Autodesk Inventor part; units mm, degrees
ref_plane "YZ Plane" through (0, 0, 0) normal (1, 0, 0) x (0, 1, 0)
ref_plane "XZ Plane" through (0, 0, 0) normal (0, 1, 0) x (-1, 0, 0)
ref_plane "XY Plane" through (0, 0, 0) normal (0, 0, 1) x (1, 0, 0)
sketch "Sketch1" plane through (0, 0, 0) normal (0, 0, 1) x (1, 0, 0)
  line L0 (0, 0) -> (66.675, 0)
  line L1 (66.675, 0) -> (66.675, 12.7)
  line L2 (66.675, 12.7) -> (0, 12.7)
  line L3 (0, 12.7) -> (0, 0)
  dimension "d0" = 66.675
  dimension "d1" = 12.7
extrude "Extrusion1" add sketch "Sketch1" along normal blind 5.08
fillet "Fillet1" radius 0.635 4 edges at (33.3375, 12.7, 0) (66.675, 6.35, 0) (33.3375, 0, 0) (0, 6.35, 0)
fillet "Fillet2" radius 0.635 8 edges at (66.489, 12.514, 0.186) (66.675, 12.7, 2.8575) (66.489, 0.186, 0.186) (66.675, 0, 2.8575) (0.186, 12.514, 0.186) (0, 12.7, 2.8575) (0.186, 0.186, 0.186) (0, 0, 2.8575)
sketch "Sketch2" plane through (0, 0, 5.08) normal (0, 0, 1) x (1, 0, 0)
  line L0 (9.525, 12.6996) -> (57.15, 12.6996)
  line L1 (57.15, 12.6996) -> (57.15, -0.0004)
  line L2 (57.15, -0.0004) -> (9.525, -0.0004)
  line L3 (9.525, -0.0004) -> (9.525, 12.6996)
  line L4 (66.675, 0.635) -> (66.675, 12.065)
  point P0 (0, 0)
  dimension "d6" = 47.625
  dimension "d7" = 12.7
  dimension "d8" = 9.525
extrude "Extrusion2" cut sketch "Sketch2" against normal blind 1.905
sketch "Sketch3" plane through (9.525, 12.6996, 5.08) normal (0, -1, 0) x (1, 0, 0)
  line L0 (0, -1.905) -> (0, 0)
  line L1 (47.625, -1.905) -> (0, -1.905)
  line L2 (0, 0) -> (47.625, 0)
  line L3 (47.625, 0) -> (47.625, -1.905)
  line L4 (47.625, -1.905) -> (0, -1.905)
  line L5 (0, -1.905) -> (0, 0)
  point P0 (-9.525, -5.08)
extrude "Extrusion3" cut sketch "Sketch3" against normal blind 0.635
sketch "Sketch4" plane through (0, 0, 5.08) normal (0, 0, 1) x (1, 0, 0)
  line L0 (0.635, 0.635) -> (66.04, 0.635)
  line L1 (58.42, 11.43) -> (59.69, 11.43)
  line L2 (59.69, 11.43) -> (59.69, 1.27)
  line L3 (59.69, 1.27) -> (58.42, 1.27)
  line L4 (58.42, 1.27) -> (58.42, 11.43)
  line L5 (66.04, 12.7) -> (0.635, 12.7)
  line L6 (57.15, 12.7) -> (57.15, 0)
  line L7 (57.15, 0) -> (66.04, 0)
  point P0 (0, 0)
  point P1 (53.975, 6.9846)
  dimension "d13" = 1.27
  dimension "d23" = 1.27
  dimension "d24" = 1.27
  dimension "d42" = 1.27
sketch "Sketch5" plane through (0, 0, 5.08) normal (0, 0, 1) x (1, 0, 0)
  line L0 (66.04, 12.065) -> (0.635, 12.065)
  line L1 (0.635, 0.635) -> (66.04, 0.635)
  line L2 (58.42, 11.43) -> (64.77, 11.43)
  line L3 (64.77, 11.43) -> (64.77, 1.27)
  line L4 (64.77, 1.27) -> (58.42, 1.27)
  line L5 (58.42, 1.27) -> (58.42, 11.43)
  line L6 (57.15, 12.7) -> (57.15, 0)
  line L7 (66.04, 12.7) -> (57.15, 12.7)
  line L8 (57.15, 0) -> (66.04, 0)
  point P0 (0, 0)
  point P1 (53.975, 6.9846)
  dimension "d14" = 6.35
  dimension "d25" = 1.27
  dimension "d43" = 1.27
  dimension "d44" = 1.27
extrude "Extrusion4" cut sketch "Sketch5" against normal through all
extrude "Extrusion5" add sketch "Sketch4" against normal blind 1.016
sketch "Sketch6" plane through (0, 0, 5.08) normal (0, 0, 1) x (1, 0, 0)
  line L0 (57.15, 12.7) -> (57.15, 0)
  line L1 (55.245, 0.635) -> (55.245, 12.065)
  line L2 (66.04, 12.065) -> (0.635, 12.065)
  line L3 (8.255, 11.43) -> (6.985, 11.43)
  line L4 (6.985, 11.43) -> (6.985, 1.27)
  line L5 (6.985, 1.27) -> (8.255, 1.27)
  line L6 (8.255, 1.27) -> (8.255, 11.43)
  line L7 (9.525, 0) -> (9.525, 12.7)
  line L8 (0.635, 0.635) -> (66.04, 0.635)
  line L9 (9.525, 12.7) -> (0.635, 12.7)
  line L10 (0.635, 0) -> (9.525, 0)
  point P0 (0, 0)
  point P1 (53.975, 6.9846)
  point P2 (6.35, 6.9846)
  dimension "d20" = 1.27
  dimension "d22" = 1.27
  dimension "d45" = 1.27
  dimension "d46" = 1.27
sketch "Sketch7" plane through (0, 0, 5.08) normal (0, 0, 1) x (1, 0, 0)
  line L0 (66.04, 12.065) -> (0.635, 12.065)
  line L1 (8.255, 11.43) -> (1.905, 11.43)
  line L2 (1.905, 11.43) -> (1.905, 1.27)
  line L3 (1.905, 1.27) -> (8.255, 1.27)
  line L4 (8.255, 1.27) -> (8.255, 11.43)
  line L5 (9.525, 0) -> (9.525, 12.7)
  line L6 (0.635, 0.635) -> (66.04, 0.635)
  line L7 (9.525, 12.7) -> (0.635, 12.7)
  line L8 (0.635, 0) -> (9.525, 0)
  point P0 (0, 0)
  point P1 (55.245, 12.065)
  point P2 (6.35, 6.9846)
  point P3 (55.245, 0.635)
  dimension "d26" = 6.35
  dimension "d28" = 1.27
  dimension "d47" = 1.27
  dimension "d48" = 1.27
extrude "Extrusion6" cut sketch "Sketch7" against normal through all
extrude "Extrusion7" add sketch "Sketch6" against normal blind 1.016 contours L6 L5 L4 L3
sketch "Sketch9" plane through (0, 0, 3.175) normal (0, 0, 1) x (1, 0, 0)
  line L0 (9.525, 0) -> (9.525, 12.7)
  line L1 (57.15, 12.7) -> (57.15, 0)
  line L2 (9.525, 12.7) -> (57.15, 12.7)
  line L3 (57.15, 12.7) -> (57.15, 11.8197)
  line L4 (57.15, 11.8197) -> (9.525, 11.8197)
  line L5 (9.525, 11.8197) -> (9.525, 12.7)
  line L6 (66.04, 0) -> (0.635, 0)
  line L7 (57.15, 0) -> (9.525, 0)
  line L8 (9.525, 0) -> (9.525, 0.889)
  line L9 (9.525, 0.889) -> (57.15, 0.889)
  line L10 (57.15, 0.889) -> (57.15, 0)
  point P0 (0, 0)
  point P1 (6.35, 6.9846)
  point P2 (53.975, 6.9846)
  dimension "d35" = 47.625
  dimension "d36" = 0.889
extrude "Extrusion8" add sketch "Sketch9" along normal blind 1.27 contours L0 L9 L1 L6 | L0 L2 L1 L4
properties part number "clipFemale"
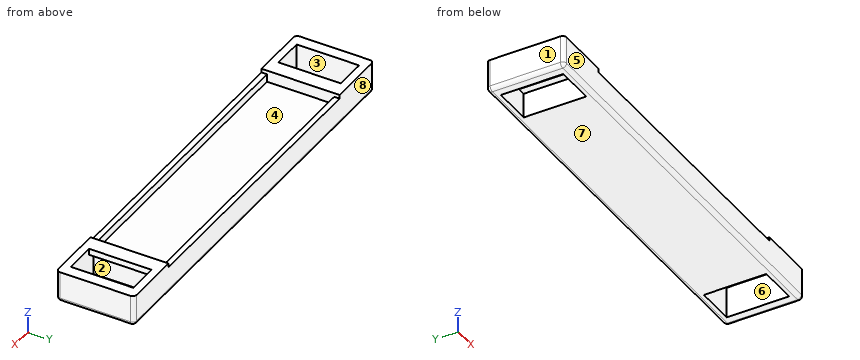
The model under review builds one solid part; all positions refer to its coordinate system, in mm. Face numbers are marked on the shaded views. A direction names the side the tool comes from. Give positions to 0.01 mm unless a question says otherwise; leave off trailing zeros. Loops run counter-clockwise (first coordinate to the right, second up) from the corner with the lowest first, then second, coordinate; pieces in that order, holes last. Notation, with made-up numbers: (-37.75, -38.75) -> (-27.75, -38.75) arc R30 ccw to (-27.75, -15.75) -> close; hole circle Ø4 at (87.5, 38.5). An arc over 180 degrees is marked (long way). Answer as a JSON object with one key per item and string values. Group by question number.
Q1. Tool access review of the marked faces 1, 2, 3 and 4: name each direction out of +Z, -Z, +X, -X, +Y, -Y from which nothing blocks a thin tool from reaching the whole face with its end or side.
Q2. Insertion check: pin 1 (4 mm diameter, centred on x = 26, y = 7, fed in from +Z) (3 decimals); pin 2 (1 mm diameter, centred on x = 23.5, y = 0.5, fed in from +Z) (3 decimals). Each pin has a flat end and moves straight along its axis. Give the tip position at first contact, or say it passes through.
Q3. Take a section at C-C (x = 13.5). Write out the cut boundary in (y, z) (3 decimals), plus the area to 3 significant figures.
Q4. Draft analysis for pull direction Y (two halves, no side actions). For the marked faces 5, 6, 7 and 8, state which applies: pulls with the +Y half, pulls with the -Y half, needs draft (parallel to the pull), parting line crosses it, or undercut.
Q5. Take a section at A-A (y = 9). Write out the cut boundary in (x, z) (3 decimals), plus the area to 3 significant figures.
Q6. Wall thickness on line 1 along X through (y, z) = (3.25, 3.25) (3 decimals); line 2 along X through (y, z) = (6, 4.4) (3 decimals); line 3 along Y through (x, z) = (63, 4): over which ranges is each line inside the solid? List them lowest first.
Q7. Take a section at B-B (z = 1.95). Write out the cut boundary in (x, y) (3 decimals).
Answer below:
{
 "1": {"face 1": "+Z, -Z, -X, +Y, -Y", "face 2": "-Z", "face 3": "+Z, -Z", "face 4": "+Z"},
 "2": {"pin 1": "stops at z = 3.175", "pin 2": "stops at z = 4.445"},
 "3": {"outline": "(0, 0.635) arc R0.635 ccw to (0.635, 0) -> (12.065, 0) arc R0.635 ccw to (12.7, 0.635) -> (12.7, 4.445) -> (11.82, 4.445) -> (11.82, 3.175) -> (0.889, 3.175) -> (0.889, 4.445) -> (0, 4.445) -> close", "area": "42.4 mm2"},
 "4": {"face 5": "pulls with the -Y half", "face 6": "undercut", "face 7": "needs draft", "face 8": "pulls with the +Y half"},
 "5": {"outline": "(0, 0.635) arc R0.635 ccw to (0.635, 0) -> (1.905, 0) -> (1.905, 5.08) -> (0, 5.08) -> close; (6.985, 4.064) -> (8.255, 4.064) -> (8.255, 0) -> (58.42, 0) -> (58.42, 4.064) -> (59.69, 4.064) -> (59.69, 5.08) -> (57.15, 5.08) -> (57.15, 3.175) -> (9.525, 3.175) -> (9.525, 5.08) -> (6.985, 5.08) -> close; (64.77, 0) -> (66.04, 0) arc R0.635 ccw to (66.675, 0.635) -> (66.675, 5.08) -> (64.77, 5.08) -> close", "area": "186 mm2"},
 "6": {"line 1": "x = 0 to 1.905, 8.255 to 9.525, 57.15 to 58.42, 64.77 to 66.675", "line 2": "x = 0 to 1.905, 6.985 to 9.525, 57.15 to 59.69, 64.77 to 66.675", "line 3": "y = 0 to 1.27, 11.43 to 12.7"},
 "7": {"outline": "(0, 0.635) arc R0.635 ccw to (0.635, 0) -> (66.04, 0) arc R0.635 ccw to (66.675, 0.635) -> (66.675, 12.065) arc R0.635 ccw to (66.04, 12.7) -> (0.635, 12.7) arc R0.635 ccw to (0, 12.065) -> close; hole (1.905, 1.27) -> (8.255, 1.27) -> (8.255, 11.43) -> (1.905, 11.43) -> close; hole (58.42, 1.27) -> (64.77, 1.27) -> (64.77, 11.43) -> (58.42, 11.43) -> close"}
}
